from build123d import *

# Parameters (mm, degrees)
MODEL_R                 = 1.5
MODEL_W                 = 3
MODEL_H                 = 3
MODEL_H_2               = 9
SALIENTE_EXTRUIR1_DEPTH = 3


with BuildPart() as part:
    # Model → Saliente-Extruir1 (new body)
    with BuildSketch(Plane.XY):
        with BuildLine():
            Line((14.191843711, 239.031739215), (14.191843711, 293.031739215))
            ThreePointArc((14.191843711, 293.031739215), (15.509863195, 296.213719731), (18.691843711, 297.531739215))
            Line((18.691843711, 297.531739215), (54.691843711, 297.531739215))
            ThreePointArc((54.691843711, 297.531739215), (57.873824226, 296.213719731), (59.191843711, 293.031739215))
            Line((59.191843711, 293.031739215), (59.191843711, 239.031739215))
            ThreePointArc((59.191843711, 239.031739215), (57.873824226, 235.8497587), (54.691843711, 234.531739215))
            Line((54.691843711, 234.531739215), (18.691843711, 234.531739215))
            ThreePointArc((18.691843711, 234.531739215), (15.509863195, 235.8497587), (14.191843711, 239.031739215))
        make_face()
        with Locations((32.191843711, 239.031739215)):
            Circle(MODEL_R, mode=Mode.SUBTRACT)
        with Locations((41.191843711, 239.031739215)):
            Circle(MODEL_R, mode=Mode.SUBTRACT)
        with Locations((32.191843711, 293.031739215)):
            Circle(MODEL_R, mode=Mode.SUBTRACT)
        with Locations((41.191843711, 293.031739215)):
            Circle(MODEL_R, mode=Mode.SUBTRACT)
        with Locations((50.191843711, 275.031739215)):
            Circle(MODEL_R, mode=Mode.SUBTRACT)
        with Locations((23.191843711, 275.031739215)):
            Circle(MODEL_R, mode=Mode.SUBTRACT)
        with Locations((18.691843711, 239.031739215)):
            Rectangle(MODEL_W, MODEL_H, mode=Mode.SUBTRACT)
        with Locations((18.691843711, 248.031739215)):
            Rectangle(MODEL_W, MODEL_H, mode=Mode.SUBTRACT)
        with Locations((18.691843711, 293.031739215)):
            Rectangle(MODEL_W, MODEL_H, mode=Mode.SUBTRACT)
        with Locations((54.691843711, 239.031739215)):
            Rectangle(MODEL_W, MODEL_H, mode=Mode.SUBTRACT)
        with Locations((54.691843711, 248.031739215)):
            Rectangle(MODEL_W, MODEL_H, mode=Mode.SUBTRACT)
        with Locations((54.691843711, 293.031739215)):
            Rectangle(MODEL_W, MODEL_H, mode=Mode.SUBTRACT)
        with Locations((45.691843711, 239.031739215)):
            Rectangle(MODEL_W, MODEL_H, mode=Mode.SUBTRACT)
        with Locations((45.691843711, 293.031739215)):
            Rectangle(MODEL_W, MODEL_H, mode=Mode.SUBTRACT)
        with Locations((18.691843711, 266.031739215)):
            Rectangle(MODEL_W, MODEL_H, mode=Mode.SUBTRACT)
        with Locations((18.691843711, 284.031739215)):
            Rectangle(MODEL_W, MODEL_H, mode=Mode.SUBTRACT)
        with Locations((54.691843711, 266.031739215)):
            Rectangle(MODEL_W, MODEL_H, mode=Mode.SUBTRACT)
        with Locations((54.691843711, 284.031739215)):
            Rectangle(MODEL_W, MODEL_H, mode=Mode.SUBTRACT)
        with Locations((36.691843711, 239.031739215)):
            Rectangle(MODEL_W, MODEL_H, mode=Mode.SUBTRACT)
        with Locations((36.691843711, 293.031739215)):
            Rectangle(MODEL_W, MODEL_H, mode=Mode.SUBTRACT)
        with Locations((27.691843711, 239.031739215)):
            Rectangle(MODEL_W, MODEL_H, mode=Mode.SUBTRACT)
        with Locations((27.691843711, 293.031739215)):
            Rectangle(MODEL_W, MODEL_H, mode=Mode.SUBTRACT)
        with Locations((18.691843711, 257.031739215)):
            Rectangle(MODEL_W, MODEL_H_2, mode=Mode.SUBTRACT)
        with Locations((54.691843711, 257.031739215)):
            Rectangle(MODEL_W, MODEL_H_2, mode=Mode.SUBTRACT)
        with Locations((18.691843711, 275.031739215)):
            Rectangle(MODEL_W, MODEL_H_2, mode=Mode.SUBTRACT)
        with Locations((54.691843711, 275.031739215)):
            Rectangle(MODEL_W, MODEL_H_2, mode=Mode.SUBTRACT)
        with BuildLine():
            Line((26.291843711, 284.881739215), (26.291843711, 244.831739215))
            ThreePointArc((26.291843711, 244.831739215), (26.43829032, 244.478185825), (26.791843711, 244.331739215))
            Line((26.791843711, 244.331739215), (46.591843711, 244.331739215))
            ThreePointArc((46.591843711, 244.331739215), (46.945397101, 244.478185825), (47.091843711, 244.831739215))
            Line((47.091843711, 244.831739215), (47.091843711, 284.881739215))
            ThreePointArc((47.091843711, 284.881739215), (46.945397101, 285.235292606), (46.591843711, 285.381739215))
            Line((46.591843711, 285.381739215), (41.691843711, 285.381739215))
            ThreePointArc((41.691843711, 285.381739215), (40.98473693, 285.674632434), (40.691843711, 286.381739215))
            Line((40.691843711, 286.381739215), (40.691843711, 288.381739215))
            ThreePointArc((40.691843711, 288.381739215), (40.398950492, 289.088845997), (39.691843711, 289.381739215))
            Line((39.691843711, 289.381739215), (33.691843711, 289.381739215))
            ThreePointArc((33.691843711, 289.381739215), (32.98473693, 289.088845997), (32.691843711, 288.381739215))
            Line((32.691843711, 288.381739215), (32.691843711, 286.381739215))
            ThreePointArc((32.691843711, 286.381739215), (32.398950492, 285.674632434), (31.691843711, 285.381739215))
            Line((31.691843711, 285.381739215), (26.791843711, 285.381739215))
            ThreePointArc((26.791843711, 285.381739215), (26.43829032, 285.235292606), (26.291843711, 284.881739215))
        make_face(mode=Mode.SUBTRACT)
    extrude(amount=SALIENTE_EXTRUIR1_DEPTH)


solid = part.part
CAD build for the part. Positions are in the model's coordinates, mm. A direction names the side the tool comes from. Round coordinates to 2 decimals unless told otherwise and drop trailing zeros. Loops run counter-clockwise (first coordinate to the right, second up) from the corner with the lowest first, then second, coordinate; pieces in that order, holes last. Notation, with made-up numbers: (68.5, 49.25) - (99.5, 49.25) arc R27 cw to (99.5, 73.25) - close; hole circle Ø5 at (15.5, 20.25). An arc over 180 degrees is marked (long way). Put each result on its own line as item: value.
1. Slice it at B-B on x = 28.5. List the corners of the cut face in (y, z).
Geometry check:
outline: (234.53, 0) - (237.53, 0) - (237.53, 3) - (234.53, 3) - close; (240.53, 0) - (244.33, 0) - (244.33, 3) - (240.53, 3) - close; (285.38, 0) - (291.53, 0) - (291.53, 3) - (285.38, 3) - close; (294.53, 0) - (297.53, 0) - (297.53, 3) - (294.53, 3) - close
2. Two-plate mould, pull along Y, no slides. Class faces 1 (the flat face through (53.192, 275, 1)), 2 (the flat face through (14.192, 266, 1)), 3 (the flat face through (28, 294.532, 1)): released by +Y, released by -Y, zero draft, split by the parting line, or undercut.
Geometry check:
face 1: undercut
face 2: zero draft
face 3: undercut
3. Slice it at C-C on x = 49.5. List the corners of the cut face in (y, z), and give its area (3 significant figures).
Geometry check:
outline: (234.53, 0) - (273.7, 0) - (273.7, 3) - (234.53, 3) - close; (276.36, 0) - (297.53, 0) - (297.53, 3) - (276.36, 3) - close
area: 181 mm²
4. 3-axis set-ups, long thin cutter, end or side, ignore diameter. For faces 4 (the flat face through (52, 266, 3)), 5 (the flat face through (53.192, 239, 1)): which of +Z, -Z, +X, -X, +Y, -Y reach the whole face in a straight line?
Geometry check:
face 4: +Z, +X, -X, +Y, -Y
face 5: +Z, -Z
5. Wall check: line 1 (Y direction, x = 29, z = 0.8); line 2 (Y direction, x = 36, z = 1.9); line 3 (X direction, y = 278, z = 0.55). Give the ranges that are in metal, low to high.
Geometry check:
line 1: 234.53 to 237.53, 240.53 to 244.33, 285.38 to 291.53, 294.53 to 297.53
line 2: 234.53 to 237.53, 240.53 to 244.33, 289.38 to 291.53, 294.53 to 297.53
line 3: 14.19 to 17.19, 20.19 to 26.29, 47.09 to 53.19, 56.19 to 59.19
6. Slice it at A-A on y = 266.5. List the corners of the cut face in (x, z).
Geometry check:
outline: (14.19, 0) - (17.19, 0) - (17.19, 3) - (14.19, 3) - close; (20.19, 0) - (26.29, 0) - (26.29, 3) - (20.19, 3) - close; (47.09, 0) - (53.19, 0) - (53.19, 3) - (47.09, 3) - close; (56.19, 0) - (59.19, 0) - (59.19, 3) - (56.19, 3) - close
7. Slice it at D-D on z = 1.7. Give the number of separate pieces and of enclosed holes in the cut face, and give its area (3 significant figures).
Geometry check:
separate pieces: 1
enclosed holes: 27
area: 1,640 mm²
